from build123d import *

# Parameters (mm, degrees)
BASE_FLANGE1_DEPTH = 5


# Sheet-metal steps are written as plain solids
with BuildPart() as part:
    # Sketch1 → Base-Flange1 (new, symmetric)
    with BuildSketch(Plane.XY):
        with BuildLine():
            Line((-10.606601718, 26.893398282), (-2.51490971, 34.98509029))
            ThreePointArc((-2.51490971, 34.98509029), (-0.909430767, 35.304439907), (0, 33.94338058))
            Line((0, 33.94338058), (0, 0.7366))
            ThreePointArc((0, 0.7366), (0.215745145, 0.215745145), (0.7366, 0))
            Line((0.7366, 0), (20, 0))
            ThreePointArc((20, 0), (29.75, 9.75), (20, 19.5))
            ThreePointArc((20, 19.5), (19, 20.5), (20, 21.5))
            ThreePointArc((20, 21.5), (26.298801772, 30.676436942), (15.471512501, 33.255527043))
            Line((15.471512501, 33.255527043), (14.97733711, 33.801759816))
            ThreePointArc((14.97733711, 33.801759816), (26.986164348, 30.94122412), (20, 20.7634))
            ThreePointArc((20, 20.7634), (19.7366, 20.5), (20, 20.2366))
            ThreePointArc((20, 20.2366), (30.4866, 9.75), (20, -0.7366))
            Line((20, -0.7366), (0.7366, -0.7366))
            ThreePointArc((0.7366, -0.7366), (-0.30510971, -0.30510971), (-0.7366, 0.7366))
            Line((-0.7366, 0.7366), (-0.7366, 33.94338058))
            ThreePointArc((-0.7366, 33.94338058), (-1.191315384, 34.623910244), (-1.994054855, 34.464235435))
            Line((-1.994054855, 34.464235435), (-10.085746863, 26.372543427))
            Line((-10.085746863, 26.372543427), (-10.606601718, 26.893398282))
        make_face()
    extrude(amount=BASE_FLANGE1_DEPTH, both=True)


solid = part.part
Read the model definition and answer for the solid it produces. Units are mm, in the model's axes. A direction names the side the tool comes from. Give positions to 0.01 mm unless a question says otherwise; leave off trailing zeros. Write each loop counter-clockwise with the first axis right and the second up, starting at its lowest first coordinate (ties: lowest second). Pieces come first, ordered by that corner, then holes. Notation, with made-up numbers: (71.5, 6.25) - (96.5, 6.25) arc R12 ccw to (96.5, 27.25) - close; hole circle Ø5 at (80.5, 67). An arc over 180 degrees is marked (long way). Use CSV: the item, a comma, the result in double quotes. Start each with the question number.
Item 1: The part is cut by section A-A, the plane y = 9.75. Give the vertices of the cut face in (x, z), and give its area (3 significant figures).
Item 2: Consider line 1 (Y direction, x = 20, z = 2.25); line 2 (Y direction, x = 21, z = 1.25); line 3 (X direction, y = 25, z = -3.5). Determine where each line is inside the solid, lowest interval first.
Item 3: The part is cut by section C-C, the plane z = 3.5. Give the vertices of the cut face in (x, y).
Item 4: For faces 1 (the cylindrical face through (29.748, 9.536, 0.07)), 2 (the flat face through (0, 18, 0)), 3 (the flat face through (-0.737, 17, 0)), 4 (the cylindrical face through (30.484, 9.981, 0.07)), determine the directions among +Z, -Z, +X, -X, +Y, -Y from which every point of the face is accessible in a straight line to the end or side of a thin tool.
Item 5: The part is cut by section B-B, the plane x = 22.5. Give the vertices of the cut face in (y, z), and give its area (3 significant figures).
Item 6: The part is cut by section D-D, the plane y = 28.25. Give the vertices of the cut face in (x, z).
Item 7: Flat-ended cylindrical pins translate along their axes: P1, Ø2, axis at y = 9.5, z = 1, coming from the -X side; P2, Ø3, axis at y = 25.5, z = -1, coming from the +X side; P3, Ø6, axis at y = 27, z = -2.5, coming from the +X side. Find the tip coordinate at first contact, or state that the pin passes through.
Taken from the geometry:
1,outline,"(-0.74, -5) - (0, -5) - (0, 5) - (-0.74, 5) - close; (29.75, -5) - (30.49, -5) - (30.49, 5) - (29.75, 5) - close"
1,area,"14.7 mm2"
2,line 1,"-0.74 to 0, 19.5 to 20.24, 20.76 to 21.5, 35 to 35.74"
2,line 2,"-0.69 to 0.05, 19.45 to 20.19, 20.83 to 21.57, 34.93 to 35.67"
2,line 3,"-0.74 to 0, 25.92 to 26.74"
3,outline,"(-10.61, 26.89) - (-10.09, 26.37) - (-1.99, 34.46) arc R0.74 cw to (-0.74, 33.94) - (-0.74, 0.74) arc R1.47 ccw to (0.74, -0.74) - (20, -0.74) arc R10.49 ccw to (20, 20.24) arc R0.26 cw to (20, 20.76) arc R7.49 ccw (long way) to (14.98, 33.8) - (15.47, 33.26) arc R6.75 cw (long way) to (20, 21.5) arc R1 ccw to (20, 19.5) arc R9.75 cw to (20, 0) - (0.74, 0) arc R0.74 cw to (0, 0.74) - (0, 33.94) arc R1.47 ccw to (-2.51, 34.99) - close"
4,face 1,"+Z, -Z"
4,face 2,"+Z, -Z, +Y"
4,face 3,"+Z, -Z, -Y"
4,face 4,"+Z, -Z, +X"
5,outline,"(-0.43, -5) - (0.33, -5) - (0.33, 5) - (-0.43, 5) - close; (19.17, -5) - (19.93, -5) - (19.93, 5) - (19.17, 5) - close; (21.19, -5) - (21.98, -5) - (21.98, 5) - (21.19, 5) - close; (34.52, -5) - (35.31, -5) - (35.31, 5) - (34.52, 5) - close"
5,area,"30.9 mm2"
6,outline,"(-9.25, -5) - (-8.21, -5) - (-8.21, 5) - (-9.25, 5) - close; (-0.74, -5) - (0, -5) - (0, 5) - (-0.74, 5) - close; (26.75, -5) - (27.49, -5) - (27.49, 5) - (26.75, 5) - close"
7,P1,"x = -0.74"
7,P2,"x = 27.38"
7,P3,"x = 27.49"
